Work out the finished part from the listing and answer in its coordinate system (mm). A direction names the side the tool comes from. Coordinates: 2 decimals unless noted, no trailing zeros. Order: outer loops, then holes, each group sorted by start corner. A loop starts at its lowest first (then second) coordinate and runs counter-clockwise, first axis right, second up.
```python
from build123d import *

# Parameters (mm, degrees)
F0_W           = 153.5
F0_H           = 82
F1_DEPTH       = 2
F2_W           = 15
F2_H           = 26
F2_W_2         = 14.5
F2_H_2         = 14.5
F3_DEPTH       = 2.001
F4_R           = 2
F5_DEPTH       = 2
F6_R           = 1.99999
F7_W           = 24
F7_H           = 35
F7_W_2         = 22
F7_H_2         = 33
F8_DEPTH       = 1
F10_R          = 4.6
F10_R_2        = 2.6
F11_DEPTH      = 4
F12_R          = 2.6
F13_DEPTH      = 4.001
F14_W          = 2
F14_H          = 35
F15_DEPTH      = 2
F15_DEPTH_BACK = 1.5
F16_R          = 1
F17_R          = 3


# Not quite as in the source:
# - a fillet or chamfer is up to 0.001 mm smaller than in the source, because OpenCascade refuses the exact size
# - a feature names something its author has since deleted; it is built from what else it names


with BuildPart() as f1:
    # F0 (on Top) → F1 (new body)
    with BuildSketch(Plane.XY):
        Rectangle(F0_W, F0_H)
    extrude(amount=F1_DEPTH)

    # F2 (on face) → F3 (cut, through all)
    with BuildSketch(Plane.XY.offset(2)):
        with Locations((44.25, 13)):
            Rectangle(F2_W, F2_H)
        with Locations((-48.75, 13)):
            Rectangle(F2_W_2, F2_H_2)
    extrude(amount=-F3_DEPTH, mode=Mode.SUBTRACT)

    # F4 (on face) → F5 (join)
    with BuildSketch(Plane.XY.offset(2)):
        with Locations((-16.25, 13)):
            Circle(F4_R)
    extrude(amount=F5_DEPTH)

    # F6 (radius 2 in the source; OpenCascade refuses exactly that, so slightly less here)
    f6_edges = [f1.edges().sort_by_distance(p)[0] for p in [
        (-18.25, 13, 4),
    ]]
    fillet(f6_edges, radius=F6_R)

    # F7 (on face) → F8 (cut)
    with BuildSketch(Plane.XY.offset(2)):
        with Locations((-48.75, 13)):
            Rectangle(F7_W, F7_H)
        with Locations((-48.75, 13)):
            Rectangle(F7_W_2, F7_H_2, mode=Mode.SUBTRACT)
    extrude(amount=-F8_DEPTH, mode=Mode.SUBTRACT)

    # F10 (on offset) → F11 (join)
    with BuildSketch(Plane.XY.offset(4)):
        with Locations((-74.75, 39)):
            Circle(F10_R)
        with Locations((-74.75, 39)):
            Circle(F10_R_2, mode=Mode.SUBTRACT)
        with Locations((74.75, 39)):
            Circle(F10_R)
        with Locations((74.75, 39)):
            Circle(F10_R_2, mode=Mode.SUBTRACT)
        with Locations((-74.75, -39)):
            Circle(F10_R)
        with Locations((-74.75, -39)):
            Circle(F10_R_2, mode=Mode.SUBTRACT)
        with Locations((74.75, -39)):
            Circle(F10_R)
        with Locations((74.75, -39)):
            Circle(F10_R_2, mode=Mode.SUBTRACT)
    extrude(amount=-F11_DEPTH)

    # F12 (on face) → F13 (cut, through all)
    with BuildSketch(Plane.XY.offset(4)):
        with Locations((-74.75, 39)):
            Circle(F12_R)
        with Locations((74.75, 39)):
            Circle(F12_R)
        with Locations((-74.75, -39)):
            Circle(F12_R)
        with Locations((74.75, -39)):
            Circle(F12_R)
    extrude(amount=-F13_DEPTH, mode=Mode.SUBTRACT)

    # F14 (on offset) → F15 (join, two sides)
    with BuildSketch(Plane.XY.offset(4)) as f15_sk:
        with Locations((-67.35, 13)):
            Rectangle(F14_W, F14_H)
    extrude(amount=-F15_DEPTH)
    extrude(f15_sk.sketch, amount=F15_DEPTH_BACK)

    # F16
    f16_edges = [f1.edges().sort_by_distance(p)[0] for p in [
        (-66.35, -4.5, 3.75),
        (-66.35, 30.5, 3.75),
    ]]
    fillet(f16_edges, radius=F16_R)

    # F17
    f17_edges = [f1.edges().sort_by_distance(p)[0] for p in [
        (-56, 20.25, 1),
        (-41.5, 5.75, 1),
        (-56, 5.75, 1),
        (-41.5, 20.25, 1),
    ]]
    fillet(f17_edges, radius=F17_R)


solid = f1.part
```
1. The part is cut by section D-D (x = 40.5). Determine the outline of the cut face in (y, z), plus the area to 3 significant figures.
2. Consider probe 1 along Y at (x, z) = (74.75, 3.1); probe 2 along X at (y, z) = (0.5, 1.15); probe 3 along Y at (x, z) = (-74.75, 1.15). Determine where each line is inside the solid, lowest interval first.
3. For faces 1 (the cylindrical face through (-42.4, 6.61, 0.99)), 2 (the cylindrical face through (77.22, 42.88, 2.03)), 3 (the flat face through (77, 37, 4)), determine the directions among +Z, -Z, +X, -X, +Y, -Y from which every point of the face is accessible in a straight line to the end or side of a thin tool.
4. The part is cut by section C-C (y = -39). Determine the outline of the cut face in (x, z).
5. The mould has two halves that part along X. Classify faces 4 (the flat face through (77, -41, 4)), 5 (the flat face through (-68.35, 13, 4)), 6 (the cylindrical face through (-42.4, 19.39, 0.99)): released by +X, released by -X, zero draft, split by the parting line, or undercut.
6. The part is cut by section B-B (x = -74.75). Determine the outline of the cut face in (y, z), plus the area to 3 significant figures.
7. Flat-ended cylindrical pins translate along their axes: pin 1 (8 mm diameter, centred on x = 38.5, y = -33, fed in from +Z); pin 2 (0.6 mm diameter, centred on y = 3.5, z = 1, fed in from -X); pin 3 (7.5 mm diameter, centred on x = 72.5, y = 41, fed in from +Z); pin 4 (2 mm diameter, centred on x = -60.5, y = 33.5, fed in from -Z). Find the tip coordinate at first contact, or state that the pin passes through.
8. The part is cut by section A-A (y = 1.5). Determine the outline of the cut face in (x, z).
Worked out:
1. outline: (-41, 0) - (0, 0) - (0, 2) - (-41, 2) - close; (26, 0) - (41, 0) - (41, 2) - (26, 2) - close
1. area: 112 mm2
2. probe 1: y = -43.6 to -41.6, -36.4 to -34.4, 34.4 to 36.4, 41.6 to 43.6
2. probe 2: x = -76.75 to -60.75, -59.75 to -37.75, -36.75 to 36.75, 51.75 to 76.75
2. probe 3: y = -43.6 to -41.6, -36.4 to 36.4, 41.6 to 43.6
3. face 1: +Z, -Z
3. face 2: +Z
3. face 3: +Z, +X, -X, +Y, -Y
4. outline: (-79.35, 0) - (-77.35, 0) - (-77.35, 4) - (-79.35, 4) - close; (-72.15, 0) - (72.15, 0) - (72.15, 4) - (70.15, 4) - (70.15, 2) - (-70.15, 2) - (-70.15, 4) - (-72.15, 4) - close; (77.35, 0) - (79.35, 0) - (79.35, 4) - (77.35, 4) - close
5. face 4: zero draft
5. face 5: released by -X
5. face 6: undercut
6. outline: (-43.6, 0) - (-41.6, 0) - (-41.6, 4) - (-43.6, 4) - close; (-36.4, 0) - (36.4, 0) - (36.4, 4) - (34.4, 4) - (34.4, 2) - (-34.4, 2) - (-34.4, 4) - (-36.4, 4) - close; (41.6, 0) - (43.6, 0) - (43.6, 4) - (41.6, 4) - close
6. area: 170 mm2
7. pin 1: stops at z = 2
7. pin 2: stops at x = -76.75
7. pin 3: stops at z = 4
7. pin 4: stops at z = 0
8. outline: (-76.75, 0) - (36.75, 0) - (36.75, 2) - (-36.75, 2) - (-36.75, 1) - (-37.75, 1) - (-37.75, 2) - (-59.75, 2) - (-59.75, 1) - (-60.75, 1) - (-60.75, 2) - (-66.35, 2) - (-66.35, 5.5) - (-68.35, 5.5) - (-68.35, 2) - (-76.75, 2) - close; (51.75, 0) - (76.75, 0) - (76.75, 2) - (51.75, 2) - close
